Check sheet for the modelled part. Datum: model origin and axes. Units: mm. Face numbers are marked on the shaded views. A direction names the side the tool comes from. Coordinates: 2 decimals unless noted, no trailing zeros. Write each loop counter-clockwise with the first axis right and the second up, starting at its lowest first coordinate (ties: lowest second). Pieces come first, ordered by that corner, then holes. Notation, with made-up numbers: M -24.5,-4.5 L 12.5,-4.5 A14 ccw 12.5,5.5 Z; hole C -32,43 d8. An arc over 180 degrees is marked long. Answer as CSV lines item,"result".
from build123d import *

# Parameters (mm, degrees)
BOSS_EXTRUDE2_DEPTH = 25.4
SKETCH5_R           = 3.048
CUT_EXTRUDE1_DEPTH  = 27.387718251
FILLET1_R           = 0.254


with BuildPart() as part:
    # Sketch4 → Boss-Extrude2 (new body)
    with BuildSketch(Plane(origin=(0, 0, 0), x_dir=(1, 0, 0), z_dir=(0, 1, 0))):
        with BuildLine():
            Line((1.27, 5.08), (-1.27, 5.08))
            Line((-1.27, 5.08), (-1.27, 3.860465775))
            ThreePointArc((-1.27, 3.860465775), (-2.032, 3.519527241), (-2.708261432, 3.03008515))
            Line((-2.708261432, 3.03008515), (-3.764409051, 3.639852263))
            Line((-3.764409051, 3.639852263), (-5.034409051, 1.440147737))
            Line((-5.034409051, 1.440147737), (-3.978261432, 0.830380625))
            ThreePointArc((-3.978261432, 0.830380625), (-4.064, 0), (-3.978261432, -0.830380625))
            Line((-3.978261432, -0.830380625), (-5.034409051, -1.440147737))
            Line((-5.034409051, -1.440147737), (-3.764409051, -3.639852263))
            Line((-3.764409051, -3.639852263), (-2.708261432, -3.03008515))
            ThreePointArc((-2.708261432, -3.03008515), (-2.032, -3.519527241), (-1.27, -3.860465775))
            Line((-1.27, -3.860465775), (-1.27, -5.08))
            Line((-1.27, -5.08), (1.27, -5.08))
            Line((1.27, -5.08), (1.27, -3.860465775))
            ThreePointArc((1.27, -3.860465775), (2.032, -3.519527241), (2.708261432, -3.03008515))
            Line((2.708261432, -3.03008515), (3.764409051, -3.639852263))
            Line((3.764409051, -3.639852263), (5.034409051, -1.440147737))
            Line((5.034409051, -1.440147737), (3.978261432, -0.830380625))
            ThreePointArc((3.978261432, -0.830380625), (4.064, 0), (3.978261432, 0.830380625))
            Line((3.978261432, 0.830380625), (5.034409051, 1.440147737))
            Line((5.034409051, 1.440147737), (3.764409051, 3.639852263))
            Line((3.764409051, 3.639852263), (2.708261432, 3.03008515))
            ThreePointArc((2.708261432, 3.03008515), (2.032, 3.519527241), (1.27, 3.860465775))
            Line((1.27, 3.860465775), (1.27, 5.08))
        make_face()
    extrude(amount=BOSS_EXTRUDE2_DEPTH)

    # Sketch5 → Cut-Extrude1 (cut, through all)
    with BuildSketch(Plane(origin=(0, 25.4, 0), x_dir=(1, 0, 0), z_dir=(0, 1, 0))):
        with Locations(Location((0, 0, 0), (0, 0, 270))):
            Circle(SKETCH5_R)
    extrude(amount=-CUT_EXTRUDE1_DEPTH, mode=Mode.SUBTRACT)

    # Fillet1
    fillet1_edges = [part.edges().sort_by_distance(p)[0] for p in [
        (2.708261432, 12.7, -3.03008515),
        (3.764409051, 12.7, -3.639852263),
        (5.034409051, 12.7, -1.440147737),
        (3.978261432, 12.7, -0.830380625),
        (3.978261432, 12.7, 0.830380625),
        (5.034409051, 12.7, 1.440147737),
        (3.764409051, 12.7, 3.639852263),
        (2.708261432, 12.7, 3.03008515),
        (1.27, 12.7, 3.860465775),
        (1.27, 12.7, 5.08),
        (-1.27, 12.7, 5.08),
        (-1.27, 12.7, 3.860465775),
        (-2.708261432, 12.7, 3.03008515),
        (-3.764409051, 12.7, 3.639852263),
        (-5.034409051, 12.7, 1.440147737),
        (-3.978261432, 12.7, 0.830380625),
        (-3.978261432, 12.7, -0.830380625),
        (-5.034409051, 12.7, -1.440147737),
        (-3.764409051, 12.7, -3.639852263),
        (-2.708261432, 12.7, -3.03008515),
        (-1.27, 12.7, -3.860465775),
        (-1.27, 12.7, -5.08),
        (1.27, 12.7, -5.08),
        (1.27, 12.7, -3.860465775),
    ]]
    fillet(fillet1_edges, radius=FILLET1_R)


solid = part.part
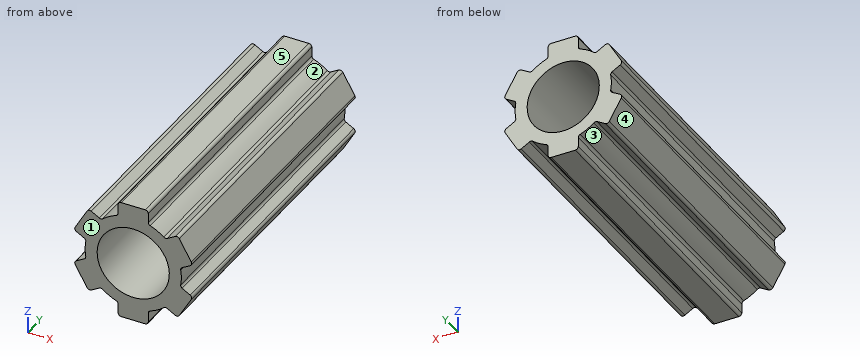
1) Section check B-B, the plane z = 0. Record the boundary of the cut face in (x, y), plus the area to 3 significant figures.
Answer key:
outline,"M -4.06,0 L -3.05,0 L -3.05,25.4 L -4.06,25.4 Z; M 3.05,0 L 4.06,0 L 4.06,25.4 L 3.05,25.4 Z"
area,"51.6 mm2"
2) Section check A-A, the plane x = 0. Record the boundary of the cut face in (y, z), plus the area to 3 significant figures.
Answer key:
outline,"M 0,-5.08 L 25.4,-5.08 L 25.4,-3.05 L 0,-3.05 Z; M 0,3.05 L 25.4,3.05 L 25.4,5.08 L 0,5.08 Z"
area,"103 mm2"
3) Section check C-C, the plane z = 4.5. Record the boundary of the cut face in (x, y), plus the area to 3 significant figures.
Answer key:
outline,"M -1.27,0 L 1.27,0 L 1.27,25.4 L -1.27,25.4 Z"
area,"64.5 mm2"
4) Tool access check on the marked faces 1 and 2. Record the directions out of +Z, -Z, +X, -X, +Y, -Y that give a thin tool (end or side, any length) a straight path to the whole face; none if there is none.
Answer key:
face 1,"+Z, -Z, +X, -X, -Y"
face 2,"+Z, +Y, -Y"
5) Depth check by flat-ended pin: P1, Ø0.9, axis at y = 7, z = -4.5, coming from the +X side; P2, Ø1.5, axis at y = 3.5, z = -0.5, coming from the -X side. Enter the tip coordinate at first touch or a pass-through.
Answer key:
P1,"stops at x = 1.27"
P2,"stops at x = -4.71"
6) Thickness scan on line 1 along X through (y, z) = (13.75, 0); line 2 along Z through (x, y) = (-4.5, 14.25); line 3 along Z through (x, y) = (-2.75, 23.5). Record the ranges inside material, lowest first.
Answer key:
line 1,"x = -4.06 to -3.05, 3.05 to 4.06"
line 2,"z = -2.37 to -1.13, 1.13 to 2.37"
line 3,"z = -3.09 to -1.31, 1.31 to 3.09"
7) Mould release check, pull along X, two halves, no side actions. Record for the marked faces 3, 4 and 5: pulls with the +X half, pulls with the -X half, needs draft (parallel to the pull), parting line crosses it, or undercut.
Answer key:
face 3,"undercut"
face 4,"pulls with the -X half"
face 5,"needs draft"
